Design review of the part built by this model. Coordinates are the model's own, in mm. Round coordinates to 2 decimals unless told otherwise and drop trailing zeros. Use a Markdown table: item, result. Add a question column.
from build123d import *

# Parameters (mm, degrees)
F0_W     = 575.685959
F0_H     = 1000
F1_DEPTH = 25
F3_SIZE  = 5
F4_SIZE  = 5
F5_SIZE  = 5
F6_SIZE  = 5
F8_D     = 32


with BuildPart() as f1:
    # F0 (on Top) → F1 (new body)
    with BuildSketch(Plane.XY):
        with Locations((16.41995, 372.970969)):
            Rectangle(F0_W, F0_H)
    extrude(amount=F1_DEPTH)

    # F3
    f3_edges = [f1.edges().sort_by_distance(p)[0] for p in [
        (16.419951, -127.029031, 25),
    ]]
    chamfer(f3_edges, length=F3_SIZE)

    # F4
    f4_edges = [f1.edges().sort_by_distance(p)[0] for p in [
        (304.26293, 375.470969, 25),
    ]]
    chamfer(f4_edges, length=F4_SIZE)

    # F5
    f5_edges = [f1.edges().sort_by_distance(p)[0] for p in [
        (-271.423029, 375.470969, 25),
    ]]
    chamfer(f5_edges, length=F5_SIZE)

    # F6
    f6_edges = [f1.edges().sort_by_distance(p)[0] for p in [
        (16.419951, 872.970969, 25),
    ]]
    chamfer(f6_edges, length=F6_SIZE)

    # F8 (through all)
    with Locations(Plane.XY.offset(25)):
        with Locations((64.978719, 617.952704), (70.463941, 139.750063)):
            Hole(F8_D / 2)


solid = f1.part
1. Mouldability with a two-part tool opening along X and no side actions: class faces 1 (the face through (-271.423, 366, 10)), 2 (the face through (12, 380, 0)), 3 (the face through (73.93, 124.13, 12.33)) as +X half, -X half, draft (parallel to the pull), parting line (faces both ways), or undercut.
2. To check wall thickness, follow probe 1 along X at (y, z) = (577, 23); probe 2 along X at (y, z) = (145, 10); probe 3 along X at (y, z) = (-23.5, 24.25). State the ranges of each line that lie inside material, in increasing order. Write a range as from..to.
3. Insertion check: P1, Ø1, axis at y = 760.5, z = 21.5, coming from the -X side; P2, Ø1, axis at x = 17, z = 21, coming from the +Y side; P3, Ø5, axis at x = -169, y = 707, coming from the -Z side. Each pin has a flat end and moves straight along its axis. Give the tip position at first contact, or say it passes through.
Verdict:
| question | item | result |
|---|---|---|
| 1 | face 1 | -X half |
| 1 | face 2 | draft |
| 1 | face 3 | undercut |
| 2 | probe 1 | x = -268.42..301.26 |
| 2 | probe 2 | x = -271.42..55.35, 85.58..304.26 |
| 2 | probe 3 | x = -267.17..300.01 |
| 3 | P1 | stops at x = -270.42 |
| 3 | P2 | stops at y = 872.47 |
| 3 | P3 | stops at z = 0 |
